Here's how the part is built. I have some questions about the finished solid (model axes, mm). Give positions to 0.01 mm unless a question says otherwise; leave off trailing zeros. Write each loop counter-clockwise with the first axis right and the second up, starting at its lowest first coordinate (ties: lowest second). Pieces come first, ordered by that corner, then holes. Notation, with made-up numbers: (77.25, -4) - (84.25, -4) arc R19 ccw to (84.25, 9) - close; hole circle Ø2 at (30.25, 8). An arc over 180 degrees is marked (long way). One line per item, written item: value. Start each with the question number.
1) I'm going to push flat-ended pins straight in: P1, Ø12, axis at y = -30, z = -15.5, coming from the -X side; P2, Ø23.5, axis at y = -13, z = -22.53, coming from the +X side; P3, Ø1, axis at x = 1, y = -23, coming from the -Z side; P4, Ø1, axis at x = 1, z = -8, coming from the -Y side. Where does each tip first touch, or does it pass through?
2) Please list where these lines run through material, in increasing order: L1, parallel to Y at x = 2, z = -27.5; L2, parallel to Y at x = 2.9, z = -33.5; L3, parallel to Z at x = 1.55, y = -16. Write a range as [from, to].
3) Imagine slicing it at B-B on y = 9. Write out the boundary of the cut face in (x, z) (3 decimals), plus the area to 3 significant figures.
4) Imagine slicing it at A-A on z = 0. Write out the boundary of the cut face in (x, y) (3 decimals), plus the area to 3 significant figures.
5) Imagine slicing it at D-D on y = -27. Write out the boundary of the cut face in (x, z) (1 decimal).
6) Imagine slicing it at C-C on z = -25.5. Write out the boundary of the cut face in (x, y) (3 decimals).
from build123d import *

# Parameters (mm, degrees)
SKETCH1_R           = 41
BOSS_EXTRUDE1_DEPTH = 3.175
SKETCH2_R           = 13
SKETCH2_R_2         = 2.75
CUT_EXTRUDE1_DEPTH  = 25


with BuildPart() as part:
    # Sketch1 → Boss-Extrude1 (new body)
    with BuildSketch(Plane(origin=(0, 0, 0), x_dir=(0, 0, -1), z_dir=(1, 0, 0))):
        Circle(SKETCH1_R)
    extrude(amount=BOSS_EXTRUDE1_DEPTH)

    # Sketch2 → Cut-Extrude1 (cut)
    with BuildSketch(Plane(origin=(3.175, 0, 0), x_dir=(0, 0, -1), z_dir=(1, 0, 0))):
        Circle(SKETCH2_R)
        with Locations((0, 26.01)):
            Circle(SKETCH2_R)
        with Locations((22.525320752, 13.005)):
            Circle(SKETCH2_R)
        with Locations((22.525320752, -13.005)):
            Circle(SKETCH2_R)
        with Locations((0, -26.01)):
            Circle(SKETCH2_R)
        with Locations((-22.525320752, -13.005)):
            Circle(SKETCH2_R)
        with Locations((-22.525320752, 13.005)):
            Circle(SKETCH2_R)
        with Locations((-18, 31.176914536)):
            Circle(SKETCH2_R_2)
        with Locations((18, 31.176914536)):
            Circle(SKETCH2_R_2)
        with Locations((36, 0)):
            Circle(SKETCH2_R_2)
        with Locations((18, -31.176914536)):
            Circle(SKETCH2_R_2)
        with Locations((-18, -31.176914536)):
            Circle(SKETCH2_R_2)
        with Locations((-36, 0)):
            Circle(SKETCH2_R_2)
    extrude(amount=-CUT_EXTRUDE1_DEPTH, mode=Mode.SUBTRACT)


solid = part.part
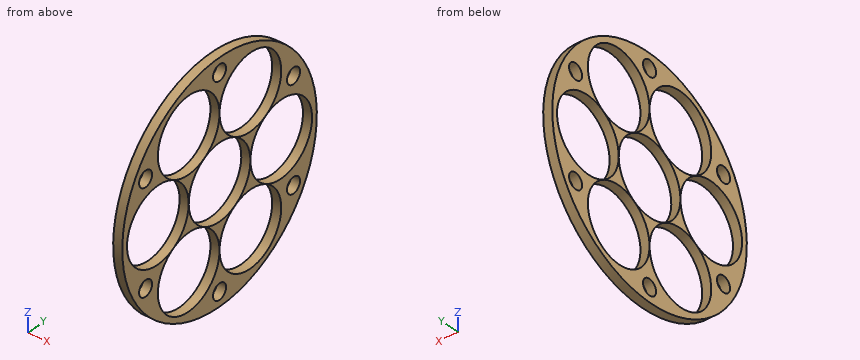
Numbers:
1. P1: x = 0
1. P2: through
1. P3: z = -34.27
1. P4: y = -40.31
2. L1: [-30.41, -25.02], [-0.99, 0.99], [25.02, 30.41]
2. L2: [-23.64, -19.97], [-6.04, -1.15], [1.15, 6.04], [19.97, 23.64]
2. L3: [-37.75, -35.18], [-9.88, -8.29], [8.29, 9.88], [35.18, 37.75]
3. outline: (0, -40) - (3.175, -40) - (3.175, -34.893) - (0, -34.893) - close; (0, -10.158) - (3.175, -10.158) - (3.175, -9.381) - (0, -9.381) - close; (0, 9.381) - (3.175, 9.381) - (3.175, 10.158) - (0, 10.158) - close; (0, 34.893) - (3.175, 34.893) - (3.175, 40) - (0, 40) - close
3. area: 37.4 mm^2
4. outline: (0, -41) - (3.175, -41) - (3.175, -39.01) - (0, -39.01) - close; (0, -13.01) - (3.175, -13.01) - (3.175, -13) - (0, -13) - close; (0, 13) - (3.175, 13) - (3.175, 13.01) - (0, 13.01) - close; (0, 39.01) - (3.175, 39.01) - (3.175, 41) - (0, 41) - close
4. area: 12.7 mm^2
5. outline: (0, -30.9) - (3.2, -30.9) - (3.2, -13) - (0, -13) - close; (0, 13) - (3.2, 13) - (3.2, 30.9) - (0, 30.9) - close
6. outline: (0, -32.105) - (3.175, -32.105) - (3.175, -25.66) - (0, -25.66) - close; (0, -0.35) - (3.175, -0.35) - (3.175, 0.35) - (0, 0.35) - close; (0, 25.66) - (3.175, 25.66) - (3.175, 32.105) - (0, 32.105) - close
